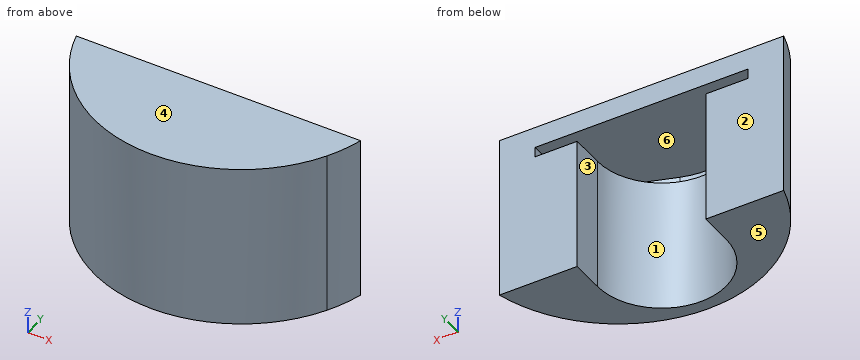
```python
from build123d import *

# Parameters (mm, degrees)
BOSS_EXTRUDE1_DEPTH = 50
CAVITY1_DEPTH       = 42.56
CAVITY1_START       = 40.52
CAVITY1_2_DEPTH     = 2.04
CAVITY1_START_2     = 41.54
CAVITY1_3_DEPTH     = 1.02
CUT_EXTRUDE1_START  = -42.56
CUT_EXTRUDE1_DEPTH  = 42.56
CUT_EXTRUDE2_DEPTH  = 80.011407404
BOSS_EXTRUDE2_DEPTH = 10
CUT_EXTRUDE3_DEPTH  = 1
SKETCH7_W           = 6.44
SKETCH7_H           = 10
BOSS_EXTRUDE3_DEPTH = 38.862
BOSS_EXTRUDE4_DEPTH = 50


# Read off the part's stored shape, not the designer's step: Cavity1
with BuildPart() as part:
    # Sketch1 → Boss-Extrude1 (new body)
    with BuildSketch(Plane.XY):
        with BuildLine():
            Line((42.035699114, -14.45), (-42.035699114, -14.45))
            ThreePointArc((-42.035699114, -14.45), (0, -44.45), (42.035699114, -14.45))
        make_face()
    extrude(amount=BOSS_EXTRUDE1_DEPTH)

    # Cavity1 outline → Cavity1 (cut)
    with BuildSketch(Plane.XY):
        with BuildLine():
            ThreePointArc((-18.145557611, -14.45), (0, -40.831), (18.145557611, -14.45))
            Line((18.145557611, -14.45), (13.723350293, -14.45))
            ThreePointArc((13.723350293, -14.45), (0, -36.782875), (-13.723350293, -14.45))
            Line((-13.723350293, -14.45), (-18.145557611, -14.45))
        make_face()
    extrude(amount=CAVITY1_DEPTH, mode=Mode.SUBTRACT)

    # Cavity1 2 outline → Cavity1 2 (cut)
    with BuildSketch(Plane.XY.offset(CAVITY1_START)):
        with BuildLine():
            Line((30.602528867, -14.45), (18.145557611, -14.45))
            ThreePointArc((18.145557611, -14.45), (0, -40.831), (-18.145557611, -14.45))
            Line((-18.145557611, -14.45), (-30.602528867, -14.45))
            ThreePointArc((-30.602528867, -14.45), (-30.998341956, -27.419452985), (-21.93, -36.7))
            Line((-21.93, -36.7), (-6.816880824, -41.760107486))
            ThreePointArc((-6.816880824, -41.760107486), (0, -42.871), (6.816880824, -41.760107486))
            Line((6.816880824, -41.760107486), (21.93, -36.7))
            ThreePointArc((21.93, -36.7), (30.998341956, -27.419452985), (30.602528867, -14.45))
        make_face()
    extrude(amount=CAVITY1_2_DEPTH, mode=Mode.SUBTRACT)

    # Cavity1 3 outline → Cavity1 3 (cut)
    with BuildSketch(Plane.XY.offset(CAVITY1_START_2)):
        with BuildLine():
            ThreePointArc((-13.723350293, -14.45), (0, -36.782875), (13.723350293, -14.45))
            Line((13.723350293, -14.45), (7.578589464, -14.45))
            ThreePointArc((7.578589464, -14.45), (0, -31.682875), (-7.578589464, -14.45))
            Line((-7.578589464, -14.45), (-13.723350293, -14.45))
        make_face()
    extrude(amount=CAVITY1_3_DEPTH, mode=Mode.SUBTRACT)

    # Sketch2 → Cut-Extrude1 (cut)
    with BuildSketch(Plane(origin=(0, 0, 0), x_dir=(-1, 0, 0), z_dir=(0, 0, -1)).offset(CUT_EXTRUDE1_START)):
        with BuildLine():
            Line((13.723350293, -14.45), (-13.723350293, -14.45))
            ThreePointArc((-13.723350293, -14.45), (0, -36.782875), (13.723350293, -14.45))
        make_face()
    extrude(amount=CUT_EXTRUDE1_DEPTH, mode=Mode.SUBTRACT)

    # Sketch4 → Cut-Extrude2 (cut, through all)
    with BuildSketch(Plane(origin=(0, 0, 0), x_dir=(-1, 0, 0), z_dir=(0, 0, -1))):
        with BuildLine():
            ThreePointArc((-42.035699114, -14.45), (-40.646415857, -17.990869296), (-38.9594982, -21.4))
            Line((-38.9594982, -21.4), (-19.431, -21.4))
            ThreePointArc((-19.431, -21.4), (-19.106937103, -17.866062319), (-18.145557611, -14.45))
            Line((-18.145557611, -14.45), (-42.035699114, -14.45))
        make_face()
        with BuildLine():
            Line((19.431, -21.4), (38.9594982, -21.4))
            ThreePointArc((38.9594982, -21.4), (40.646415857, -17.990869296), (42.035699114, -14.45))
            Line((42.035699114, -14.45), (18.145557611, -14.45))
            ThreePointArc((18.145557611, -14.45), (19.106937103, -17.866062319), (19.431, -21.4))
        make_face()
    extrude(amount=-CUT_EXTRUDE2_DEPTH, mode=Mode.SUBTRACT)

    # Sketch5 → Boss-Extrude2 (add)
    with BuildSketch(Plane(origin=(0, -21.4, 0), x_dir=(1, 0, 0), z_dir=(0, 1, 0))):
        Polygon((-32.13, -42.56), (-32.13, -40.52), (-19.431, -40.52), (-19.431, 0), (-38.9594982, 0), (-38.9594982, -50), (-19.431, -50), (-19.431, -42.56), align=None)
        Polygon((19.431, -42.56), (19.431, -50), (38.9594982, -50), (38.9594982, 0), (19.431, 0), (19.431, -40.52), (32.13, -40.52), (32.13, -42.56), align=None)
    extrude(amount=BOSS_EXTRUDE2_DEPTH)

    # Sketch6 → Cut-Extrude3 (cut)
    with BuildSketch(Plane(origin=(0, 0, 42.56), x_dir=(-1, 0, 0), z_dir=(0, 0, -1))):
        with BuildLine():
            Line((-19.431, -21.4), (-19.431, -11.4))
            Line((-19.431, -11.4), (-32.13, -11.4))
            Line((-32.13, -11.4), (-32.13, -21.4))
            ThreePointArc((-32.13, -21.4), (-29.346233629, -30.594155752), (-21.93, -36.7))
            Line((-21.93, -36.7), (-6.816880824, -41.760107486))
            ThreePointArc((-6.816880824, -41.760107486), (0, -42.871), (6.816880824, -41.760107486))
            Line((6.816880824, -41.760107486), (21.93, -36.7))
            ThreePointArc((21.93, -36.7), (29.346233629, -30.594155752), (32.13, -21.4))
            Line((32.13, -21.4), (32.13, -11.4))
            Line((32.13, -11.4), (19.431, -11.4))
            Line((19.431, -11.4), (19.431, -21.4))
            ThreePointArc((19.431, -21.4), (19.106937103, -17.866062319), (18.145557611, -14.45))
            Line((18.145557611, -14.45), (-18.145557611, -14.45))
            ThreePointArc((-18.145557611, -14.45), (-19.106937103, -17.866062319), (-19.431, -21.4))
        make_face()
    extrude(amount=-CUT_EXTRUDE3_DEPTH, mode=Mode.SUBTRACT)

    # Sketch7 → Boss-Extrude3 (add)
    with BuildSketch(Plane.ZY.offset(-19.431)):
        with Locations((46.78, -16.4)):
            Rectangle(SKETCH7_W, SKETCH7_H)
    extrude(amount=BOSS_EXTRUDE3_DEPTH)

    # Sketch8 → Boss-Extrude4 (add, through all)
    with BuildSketch(Plane(origin=(0, 0, 0), x_dir=(-1, 0, 0), z_dir=(0, 0, -1))):
        with BuildLine():
            Line((-38.9594982, -21.4), (-38.9594982, -11.4))
            Line((-38.9594982, -11.4), (-42.963269196, -11.4))
            ThreePointArc((-42.963269196, -11.4), (-41.265420808, -16.521729496), (-38.9594982, -21.4))
        make_face()
        with BuildLine():
            Line((38.9594982, -11.4), (42.963269196, -11.4))
            ThreePointArc((42.963269196, -11.4), (41.265420808, -16.521729496), (38.9594982, -21.4))
            Line((38.9594982, -21.4), (38.9594982, -11.4))
        make_face()
    extrude(amount=-BOSS_EXTRUDE4_DEPTH)


solid = part.part
```
Can you work these out from the model? Positions are in its coordinate system, mm. Face numbers are marked on the shaded views. A direction names the side the tool comes from. Give positions to 0.01 mm unless a question says otherwise; leave off trailing zeros. Order: outer loops, then holes, each group sorted by start corner. A loop starts at its lowest first (then second) coordinate and runs counter-clockwise, first axis right, second up. Notation, with made-up numbers: M 66.25,-14.75 L 77.25,-14.75 A12 ccw 77.25,1.25 Z; hole C 64,19 d11. An arc over 180 degrees is marked long. One line per item, written item: value.
1) I want a section at A-A, the plane x = -18.5. List the corners of the cut face in (y, z) for me.
Answer sheet:
outline: M -40.42,0 L -27.34,0 L -27.34,40.52 L -37.85,40.52 L -37.85,43.56 L -11.4,43.56 L -11.4,50 L -40.42,50 Z
2) On a 3-axis mill with a long thin cutter (end or side, diameter ignored), from which of +Z, -Z, +X, -X, +Y, -Y can I reach the whole of each face in a straight line? I mean the marked faces 1 and 2. Say none if no direction works.
Answer sheet:
face 1: -Z, +Y
face 2: +Z, -Z, +X, -X, +Y
3) We'd pull the mould along Z, two halves only. Please class the marked faces 3, 4, 5 and 6: released by +Z, released by -Z, zero draft, split by the parting line, or undercut.
Answer sheet:
face 3: zero draft
face 4: released by +Z
face 5: released by -Z
face 6: undercut
4) For P1, Ø6, axis at y = -16, z = 43.5, coming from the -X side; P2, Ø4, axis at x = 2.5, y = -22.5, coming from the -Z side; P3, Ø0.9, axis at y = -16, z = 42.5, coming from the +X side; P4, Ø4, axis at x = 34, y = -25.5, coming from the -Z side, each with a flat end and sliding along its axis, tell me the tip position at first contact or that it passes through.
Answer sheet:
P1: stops at x = -42.51
P2: stops at z = 43.56
P3: stops at x = 41.64
P4: stops at z = 0
5) I want a section at C-C, the plane z = 36. List the corners of the cut face in (x, y) for me.
Answer sheet:
outline: M -42.96,-11.4 A44.45 ccw 42.96,-11.4 L 19.43,-11.4 L 19.43,-21.4 A19.43 cw -19.43,-21.4 L -19.43,-11.4 Z
6) I want a section at B-B, the plane y = -25. List the corners of the cut face in (x, z) for me, plus the area to 3 significant figures.
Answer sheet:
outline: M -36.75,0 L -19.09,0 L -19.09,40.52 L -31.73,40.52 L -31.73,43.56 L 31.73,43.56 L 31.73,40.52 L 19.09,40.52 L 19.09,0 L 36.75,0 L 36.75,50 L -36.75,50 Z
area: 1,930 mm^2
7) Please list where these lines run through material, in increasing order: line 1 along Z through (x, y) = (20, -31); line 2 along Z through (x, y) = (6, -17); line 3 along X through (y, z) = (-17.5, 24.5).
Answer sheet:
line 1: z = 0 to 40.52, 43.56 to 50
line 2: z = 43.56 to 50
line 3: x = -40.86 to -19.43, 19.43 to 40.86
8) I want a section at D-D, the plane y = -14. List the corners of the cut face in (x, z) for me.
Answer sheet:
outline: M -42.19,0 L -19.43,0 L -19.43,40.52 L -32.13,40.52 L -32.13,43.56 L 32.13,43.56 L 32.13,40.52 L 19.43,40.52 L 19.43,0 L 42.19,0 L 42.19,50 L -42.19,50 Z
